Part model, mm, in its own coordinate system. Coordinates: 2 decimals unless noted, no trailing zeros. Order: outer loops, then holes, each group sorted by start corner. A loop starts at its lowest first (then second) coordinate and runs counter-clockwise, first axis right, second up.
1) Cut at B-B (x = -10). List the corners of the cut face in (y, z), and give its area (3 significant figures).
2) Cut at A-A (x = 15). List the corners of the cut face in (y, z), and give its area (3 significant figures).
3) Mould opens along X. For faces 1 (the cylindrical face through (14.2, -17.53, 1.17)), 2 (the flat face through (0, -53.213, 1)), 3 (the flat face through (21.526, -27, 1)), 4 (the cylindrical face through (10.565, -31.468, 1.207)) say: +X half, -X half, draft (parallel to the pull), parting line (faces both ways), or undercut.
4) Wall check: L1, parallel to Y at x = -14, z = 2.35; L2, parallel to Y at x = 15.5, z = 2.2; L3, parallel to X at y = -32.5, z = 1.3. Give the ranges that are in metal, low to high.
5) Pin check, flat tip, straight feed: pin 1 Ø3.5 at (x, y) = (-10.54, -20.2) entering from -Z. Stop position of the tip, or through.
```python
from build123d import *

# Parameters (mm, degrees)
SKETCH1_W             = 43.053
SKETCH1_H             = 53.213
BOSS_EXTRUDE1_DEPTH   = 2.38125
F_4_40_TAPPED_HOLE1_D = 2.2606
SKETCH5_R             = 1.583220457
SKETCH5_R_2           = 1.481870985
CUT_EXTRUDE1_DEPTH    = 3.38125


with BuildPart() as part:
    # Sketch1 → Boss-Extrude1 (new body)
    with BuildSketch(Plane.XY):
        with Locations((0, -26.6065)):
            Rectangle(SKETCH1_W, SKETCH1_H)
    extrude(amount=BOSS_EXTRUDE1_DEPTH)

    # #4-40 Tapped Hole1 (through all)
    with Locations(Plane.XY.offset(2.38125)):
        with Locations((-14.8082, -18.4804304), (14.8082, -18.4804304), (-14.8082, -34.7325696), (14.8082, -34.7325696)):
            Hole(F_4_40_TAPPED_HOLE1_D / 2)

    # Sketch5 → Cut-Extrude1 (cut, through all)
    with BuildSketch(Plane.XY.offset(2.38125)):
        with Locations((-10.538552378, -20.202865742)):
            Circle(SKETCH5_R)
        with Locations((10.758105553, -32.936949866)):
            Circle(SKETCH5_R_2)
    extrude(amount=-CUT_EXTRUDE1_DEPTH, mode=Mode.SUBTRACT)


solid = part.part
```
Geometry check:
1. outline: (-53.21, 0) - (-21.69, 0) - (-21.69, 2.38) - (-53.21, 2.38) - close; (-18.71, 0) - (0, 0) - (0, 2.38) - (-18.71, 2.38) - close
1. area: 120 mm2
2. outline: (-53.21, 0) - (-35.85, 0) - (-35.85, 2.38) - (-53.21, 2.38) - close; (-33.62, 0) - (-19.59, 0) - (-19.59, 2.38) - (-33.62, 2.38) - close; (-17.37, 0) - (0, 0) - (0, 2.38) - (-17.37, 2.38) - close
2. area: 116 mm2
3. face 1: undercut
3. face 2: draft
3. face 3: +X half
3. face 4: undercut
4. L1: y = -53.21 to -35.52, -33.94 to -19.27, -17.69 to 0
4. L2: y = -53.21 to -35.63, -33.84 to -19.37, -17.59 to 0
4. L3: x = -21.53 to 9.34, 12.17 to 21.53
5. pin 1: stops at z = 0
